```python
from build123d import *

# Parameters (mm, degrees)
F0_W     = 38.1
F0_H     = 38.1
F1_DEPTH = 38.1
F6_DEPTH = 38.1
F8_DEPTH = 38.1


with BuildPart() as f1:
    # F0 (on Front) → F1 (new body)
    with BuildSketch(Plane.XZ):
        with Locations((19.05, 19.05)):
            Rectangle(F0_W, F0_H)
    extrude(amount=F1_DEPTH)

    # F4 (on offset) → F6 (cut)
    with BuildSketch(Plane.YZ.offset(38.1)):
        Polygon((-38.1, 38.1), (-38.1, 0), (-32.075848, 0), align=None)
        Polygon((-6.35, 38.1), (-31.75, 38.1), (-26.67, 23.803649), (-21.59, 25.608752), (-16.51, 25.608752), (-11.43, 23.803649), align=None)
        Polygon((0, 38.1), (-6.35, 0), (0, 0), align=None)
        Polygon((-19.212924, 15.315445), (-25.725848, 0), (-12.7, 0), align=None)
    extrude(amount=-F6_DEPTH, mode=Mode.SUBTRACT)

    # F7 (on offset) → F8 (cut)
    with BuildSketch(Plane.XZ.offset(38.1)):
        Polygon((0, 38.1), (0, 0), (6.35, 38.1), align=None)
        Polygon((38.1, 38.1), (31.75, 38.1), (38.1, 1.456059), align=None)
        Polygon((15.274494, 11.858941), (6.35, 0), (31.75, 0), (28.007285, 11.858941), (24.076072, 6.658068), (16.915904, 6.658068), align=None)
        Polygon((31.75, 38.1), (6.35, 38.1), (18.287822, 20.289955), align=None)
    extrude(amount=-F8_DEPTH, mode=Mode.SUBTRACT)


solid = f1.part
```
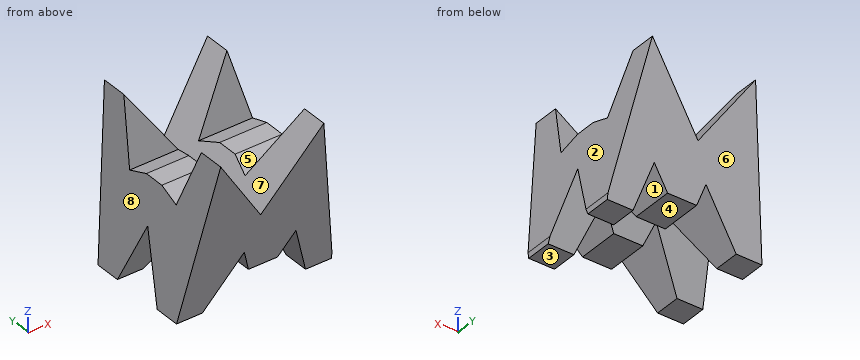
The model under review builds one solid part; all positions refer to its coordinate system, in mm. Face numbers are marked on the shaded views. A direction names the side the tool comes from. Give positions to 0.01 mm unless a question says otherwise; leave off trailing zeros. Order: outer loops, then holes, each group sorted by start corner. A loop starts at its lowest first (then second) coordinate and runs counter-clockwise, first axis right, second up. Notation, with made-up numbers: (48, 87.5) - (56, 87.5) arc R27 cw to (56, 112.5) - close; hole circle Ø7 at (45.25, -30.75). An arc over 180 degrees is marked (long way). Use CSV: the item, a comma, the result in double quotes. Start each with the question number.
Q1. We need section C-C, the plane z = 29.5. Write out the cut boundary in (x, y).
Q2. We need section B-B, the plane x = 12. Write out the cut boundary in (y, z).
Q3. The part is to be moulded in two halves that separate along X. For the marked faces 1, 2 and 3, say which applies: +X half, -X half, draft (parallel to the pull), parting line (faces both ways), or undercut.
Q4. We need section D-D, the plane y = -10. Write out the cut boundary in (x, z).
Q5. Tool access review of the marked faces 4, 5, 6, 7 and 8: name each direction out of +Z, -Z, +X, -X, +Y, -Y from which nothing blocks a thin tool from reaching the whole face with its end or side.
Q6. Clearance check with flat-ended pins moving along their axes: pin 1 Ø6 at (x, z) = (12, 22.5) entering from -Y; pin 2 Ø5.5 at (x, y) = (21.5, -8.5) entering from -Z; pin 3 Ø1.5 at (x, y) = (8.5, -19) entering from +Z. State where each tip first meets the part, or that it passes through.
Q7. We need section A-A, the plane z = 25. Write out the cut boundary in (x, y).
Q8. To check wall thickness, follow line 1 along Y through (x, z) = (9, 32.5); line 2 along Y through (x, z) = (21, 10); line 3 along X through (y, z) = (-35.5, 36.5). State the ranges of each line that lie inside material, in increasing order. Write a range as [from, to].
Outcome:
1,outline,"(4.92, -36.74) - (12.11, -36.74) - (12.11, -28.69) - (4.92, -28.69) - close; (4.92, -9.41) - (12.11, -9.41) - (12.11, -1.43) - (4.92, -1.43) - close; (25.25, -36.74) - (33.24, -36.74) - (33.24, -28.69) - (25.25, -28.69) - close; (25.25, -9.41) - (33.24, -9.41) - (33.24, -1.43) - (25.25, -1.43) - close"
2,outline,"(-36.77, 29.67) - (-33.26, 7.51) - (-22.53, 7.51) - (-19.21, 15.32) - (-15.89, 7.51) - (-5.1, 7.51) - (-1.4, 29.67) - (-9.35, 29.67) - (-11.43, 23.8) - (-16.51, 25.61) - (-21.59, 25.61) - (-26.67, 23.8) - (-28.75, 29.67) - close"
3,face 1,"undercut"
3,face 2,"+X half"
3,face 3,"draft"
4,outline,"(0, 0) - (6.35, 0) - (15.27, 11.86) - (16.92, 6.66) - (24.08, 6.66) - (28.01, 11.86) - (31.75, 0) - (38.1, 0) - (38.1, 1.46) - (33.53, 27.83) - (23.99, 27.83) - (18.29, 20.29) - (13.24, 27.83) - (4.64, 27.83) - close"
5,face 4,"-Z, +Y, -Y"
5,face 5,"+Z, +X, -X"
5,face 6,"-Z, +X, -X, +Y"
5,face 7,"+Z, +Y, -Y"
5,face 8,"+Z, -X, +Y, -Y"
6,pin 1,"stops at y = -36.11"
6,pin 2,"stops at z = 6.66"
6,pin 3,"stops at z = 25.61"
7,outline,"(4.17, -36.03) - (15.13, -36.03) - (15.13, -27.1) - (4.17, -27.1) - close; (4.17, -23.3) - (15.13, -23.3) - (15.13, -14.8) - (4.17, -14.8) - close; (4.17, -11) - (15.13, -11) - (15.13, -2.18) - (4.17, -2.18) - close; (21.85, -36.03) - (34.02, -36.03) - (34.02, -27.1) - (21.85, -27.1) - close; (21.85, -23.3) - (34.02, -23.3) - (34.02, -14.8) - (21.85, -14.8) - close; (21.85, -11) - (34.02, -11) - (34.02, -2.18) - (21.85, -2.18) - close"
8,line 1,"y = [-37.21, -29.76], [-8.34, -0.93]"
8,line 2,"y = [-33.66, -21.47], [-16.95, -4.68]"
8,line 3,"x = [6.08, 7.42], [30.54, 32.03]"
